Could you check a few things on this drawing? It's one solid part, dimensions in mm from its lowest x, y, z. A direction names the side the tool comes from. Round coordinates to 2 decimals unless told otherwise and drop trailing zeros. Order: outer loops, then holes, each group sorted by start corner. A loop starts at its lowest first (then second) coordinate and runs counter-clockwise, first axis right, second up. Notation, with made-up numbers: (15, 22.25) -> (74, 22.25) arc R22 ccw to (74, 49.25) -> close; hole circle Ø2 at (-20, 64.25). An arc over 180 degrees is marked (long way). Use a Markdown table: item, result. Add a question column.
(1) On a 3-axis mill with a long thin cutter (end or side, diameter ignored), from which of +Z, -Z, +X, -X, +Y, -Y can I reach the whole of each face in a straight line? I mean the marked faces 5 and 6. Say none if no direction works.
(2) I want a section at D-D, the plane z = 15.5. Please give me the cut outline in (x, y), then the cut area to 3 significant figures.
(3) I want a section at A-A, the plane z = 51. Please give me the cut outline in (x, y), then the cut area to 3 significant figures.
(4) I'm going to push flat-ended pins straight in: P1, Ø2, axis at x = 68, z = 70.5, coming from the -Y side; P2, Ø10, axis at x = 33, y = 35, coming from the -Z side; P3, Ø6, axis at x = 59, y = 35, coming from the -Z side. Where does each tip first touch, or does it pass through?
(5) Thinking about a two-plate mould opening in X: for the marked faces 1, 2, 3 and 4, which applies, pulls with the +X half, pulls with the -X half, needs draft (parallel to the pull), parting line crosses it, or undercut?
(6) If I drill on probe 1 along Y at (x, z) = (82.5, 36.5); probe 2 along Z at (x, y) = (60, 18) (1 decimal); probe 3 along X at (y, z) = (87, 39.5), over which ranges is the centre line in solid material (lowest first)?
(7) I want a section at B-B, the plane x = 34. Please give me the cut outline in (y, z) (1 decimal).
(8) I want a section at C-C, the plane y = 78.5. Please give me the cut outline in (x, z) (1 decimal).
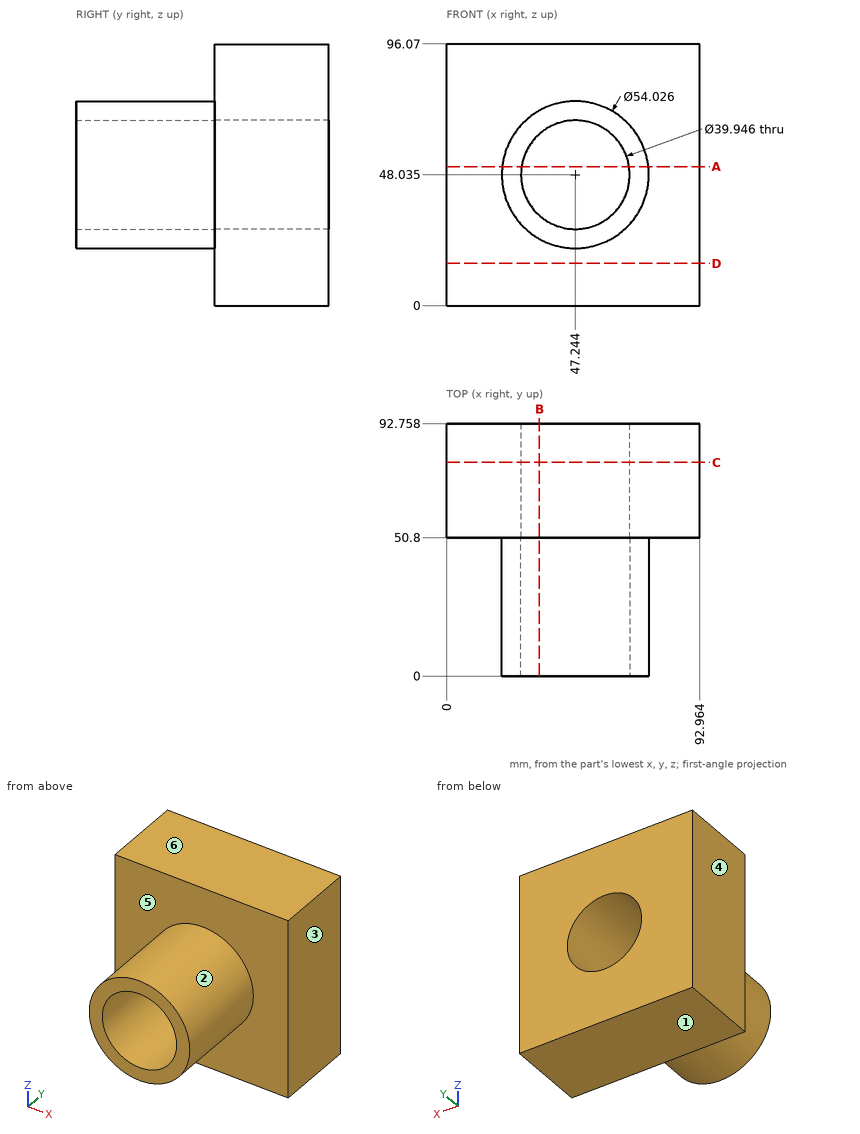
Taken from the geometry:
| question | item | result |
|---|---|---|
| 1 | face 5 | -Y |
| 1 | face 6 | +Z, +X, -X, +Y, -Y |
| 2 | outline | (0, 50.8) -> (92.96, 50.8) -> (92.96, 92.76) -> (0, 92.76) -> close |
| 2 | area | 3,900 mm2 |
| 3 | outline | (0, 50.8) -> (20.39, 50.8) -> (20.39, 0) -> (27.49, 0) -> (27.49, 92.76) -> (0, 92.76) -> close; (67, 0) -> (74.09, 0) -> (74.09, 50.8) -> (92.96, 50.8) -> (92.96, 92.76) -> (67, 92.76) -> close |
| 3 | area | 2,960 mm2 |
| 4 | P1 | stops at y = 50.8 |
| 4 | P2 | stops at z = 22.65 |
| 4 | P3 | stops at z = 22.48 |
| 5 | face 1 | needs draft |
| 5 | face 2 | parting line crosses it |
| 5 | face 3 | pulls with the +X half |
| 5 | face 4 | pulls with the -X half |
| 6 | probe 1 | y = 50.8 to 92.76 |
| 6 | probe 2 | z = 24.2 to 32.7, 63.4 to 71.8 |
| 6 | probe 3 | x = 0 to 29.19, 65.3 to 92.96 |
| 7 | outline | (0, 24.5) -> (50.8, 24.5) -> (50.8, 0) -> (92.8, 0) -> (92.8, 33.1) -> (0, 33.1) -> close; (0, 63) -> (92.8, 63) -> (92.8, 96.1) -> (50.8, 96.1) -> (50.8, 71.6) -> (0, 71.6) -> close |
| 8 | outline | (0, 0) -> (93, 0) -> (93, 96.1) -> (0, 96.1) -> close; hole circle Ø39.9 at (47.2, 48) |
